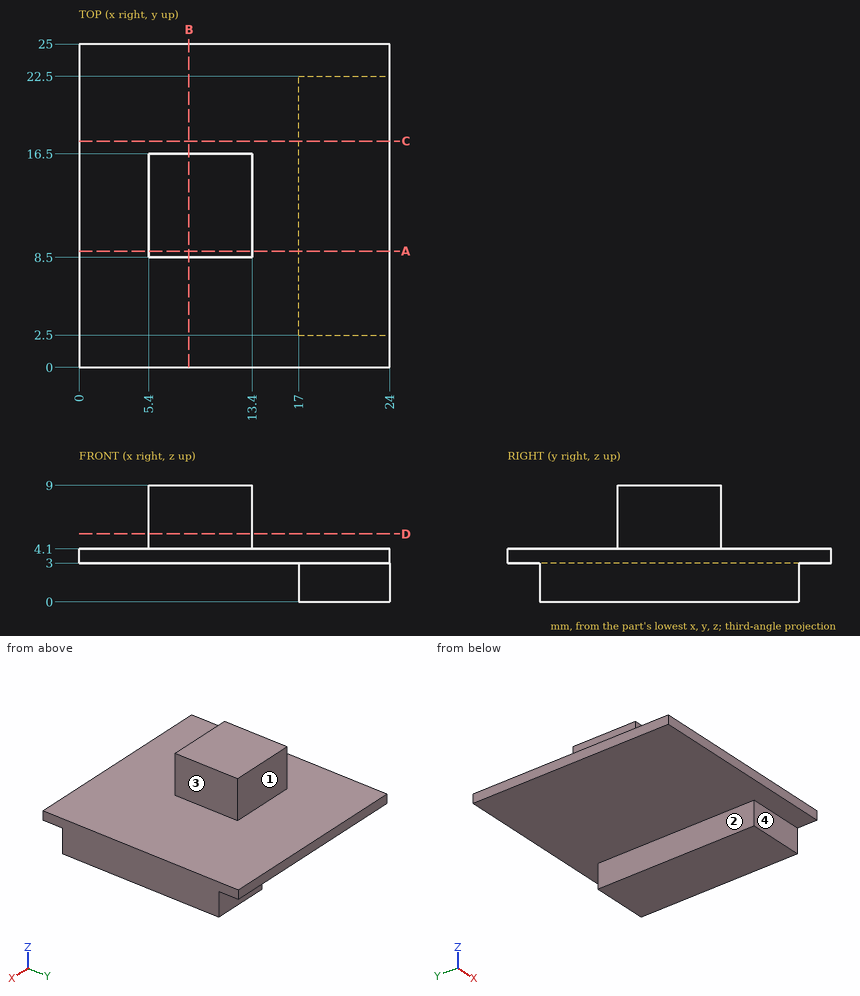
Verification items for this drawing (mm, ordinates from the low corner). A direction names the side the tool comes from. Round coordinates to 2 decimals unless told otherwise and drop trailing zeros. Order: outer loops, then holes, each group sorted by start corner. A loop starts at its lowest first (then second) coordinate and runs counter-clockwise, first axis right, second up. Notation, with made-up numbers: (0, -17.5) - (40, -17.5) arc R22 ccw to (40, 11.5) - close; hole circle Ø7 at (10.5, -11). An arc over 180 degrees is marked (long way). Use CSV: the item, a comma, the result in double quotes.
(1) Section check A-A on y = 9. Record the boundary of the cut face in (x, z).
Entries:
outline,"(0, 3) - (17, 3) - (17, 0) - (24, 0) - (24, 4.1) - (13.4, 4.1) - (13.4, 9) - (5.4, 9) - (5.4, 4.1) - (0, 4.1) - close"
(2) Section check B-B on x = 8.5. Record the boundary of the cut face in (y, z), and give its area (3 significant figures).
Entries:
outline,"(0, 3) - (25, 3) - (25, 4.1) - (16.5, 4.1) - (16.5, 9) - (8.5, 9) - (8.5, 4.1) - (0, 4.1) - close"
area,"66.7 mm^2"
(3) Thickness scan on probe 1 along Z at (x, y) = (16.5, 6.5); probe 2 along Z at (x, y) = (6.5, 10.75); probe 3 along X at (y, z) = (10, 7). Record the ranges inside material, lowest first. Write a range as from..to.
Entries:
probe 1,"3..4.1"
probe 2,"3..9"
probe 3,"5.4..13.4"
(4) Section check C-C on y = 17.5. Record the boundary of the cut face in (x, z), and give its area (3 significant figures).
Entries:
outline,"(0, 3) - (17, 3) - (17, 0) - (24, 0) - (24, 4.1) - (0, 4.1) - close"
area,"47.4 mm^2"
(5) Gauge pin test, flat ends, axial feed: pin 1 Ø4 at (y, z) = (11, 6.5) entering from -X; pin 2 Ø1.5 at (y, z) = (11, 6.5) entering from +X; pin 3 Ø2.5 at (x, z) = (9.5, 7) entering from +Y; pin 4 Ø2 at (x, z) = (12, 1.5) entering from +Y. Record the tip position at first contact, or that the pin passes through.
Entries:
pin 1,"x = 5.4"
pin 2,"x = 13.4"
pin 3,"y = 16.5"
pin 4,"through"
(6) Access from +Z, -Z, +X, -X, +Y, -Y to the whole of each face (thin tool, end or side, straight path). Record for the marked faces 1, 2, 3 and 4.
Entries:
face 1,"+Z, +X, -X, +Y"
face 2,"-Z, -X, +Y, -Y"
face 3,"+Z, +X, +Y, -Y"
face 4,"-Z, +X, -X, -Y"
(7) Section check D-D on z = 5.25. Record the boundary of the cut face in (x, y), and give its area (3 significant figures).
Entries:
outline,"(5.4, 8.5) - (13.4, 8.5) - (13.4, 16.5) - (5.4, 16.5) - close"
area,"64.0 mm^2"
